```python
from build123d import *

# Parameters (mm, degrees)
SKETCH_1_R          = 1
EXTRUDE_1_DEPTH     = 1.6
SKETCH_2_W          = 16
SKETCH_2_H          = 8
CUT_EXTRUDE_1_DEPTH = 1.6
EXTRUDE_2_DEPTH     = 1.6
SKETCH_4_W          = 1.78
SKETCH_4_H          = 8.1
CUT_EXTRUDE_2_DEPTH = 0.1
CUT_EXTRUDE_START   = 1.6
SKETCH_5_W          = 1.78
SKETCH_5_H          = 8.1
CUT_EXTRUDE_3_DEPTH = 0.1


with BuildPart() as part:
    # 草图1 → 凸台-拉伸1 (new body)
    with BuildSketch(Plane.XY):
        with BuildLine():
            Line((-14, 30), (14, 30))
            ThreePointArc((14, 30), (15.414213562, 29.414213562), (16, 28))
            Line((16, 28), (16, -28))
            ThreePointArc((16, -28), (15.414213562, -29.414213562), (14, -30))
            Line((14, -30), (-14, -30))
            ThreePointArc((-14, -30), (-15.414213562, -29.414213562), (-16, -28))
            Line((-16, -28), (-16, 28))
            ThreePointArc((-16, 28), (-15.414213562, 29.414213562), (-14, 30))
        make_face()
        with Locations((-14, 28)):
            Circle(SKETCH_1_R, mode=Mode.SUBTRACT)
        with Locations((14, 28)):
            Circle(SKETCH_1_R, mode=Mode.SUBTRACT)
    extrude(amount=EXTRUDE_1_DEPTH)

    # 草图2 → 切除-拉伸1 (cut)
    with BuildSketch(Plane.XY):
        with Locations((0, -26)):
            Rectangle(SKETCH_2_W, SKETCH_2_H)
    extrude(amount=CUT_EXTRUDE_1_DEPTH, mode=Mode.SUBTRACT)

    # 草图3 → 凸台-拉伸2 (add)
    with BuildSketch(Plane.XY):
        with BuildLine():
            Line((-13.97, 30), (13.97, 30))
            Line((13.97, 30), (13.97, 39.42))
            ThreePointArc((13.97, 39.42), (13.530660172, 40.480660172), (12.47, 40.92))
            Line((12.47, 40.92), (-12.47, 40.92))
            ThreePointArc((-12.47, 40.92), (-13.530660172, 40.480660172), (-13.97, 39.42))
            Line((-13.97, 39.42), (-13.97, 30))
        make_face()
    extrude(amount=EXTRUDE_2_DEPTH)

    # 草图4 → 切除-拉伸2 (cut)
    with BuildSketch(Plane.XY):
        with Locations((-1.27, 36.37)):
            Rectangle(SKETCH_4_W, SKETCH_4_H)
        with Locations((-3.81, 36.37)):
            Rectangle(SKETCH_4_W, SKETCH_4_H)
        with Locations((-6.35, 36.37)):
            Rectangle(SKETCH_4_W, SKETCH_4_H)
        with Locations((-8.89, 36.37)):
            Rectangle(SKETCH_4_W, SKETCH_4_H)
        with Locations((-11.43, 36.37)):
            Rectangle(SKETCH_4_W, SKETCH_4_H)
        with Locations((11.43, 36.37)):
            Rectangle(SKETCH_4_W, SKETCH_4_H)
        with Locations((8.89, 36.37)):
            Rectangle(SKETCH_4_W, SKETCH_4_H)
        with Locations((6.35, 36.37)):
            Rectangle(SKETCH_4_W, SKETCH_4_H)
        with Locations((3.81, 36.37)):
            Rectangle(SKETCH_4_W, SKETCH_4_H)
        with Locations((1.27, 36.37)):
            Rectangle(SKETCH_4_W, SKETCH_4_H)
    extrude(amount=CUT_EXTRUDE_2_DEPTH, mode=Mode.SUBTRACT)

    # 草图5 → 切除-拉伸3 (cut)
    with BuildSketch(Plane.XY.offset(CUT_EXTRUDE_START)):
        with Locations((-3.81, 36.37)):
            Rectangle(SKETCH_5_W, SKETCH_5_H)
        with Locations((-1.27, 36.37)):
            Rectangle(SKETCH_5_W, SKETCH_5_H)
        with Locations((-11.43, 36.37)):
            Rectangle(SKETCH_5_W, SKETCH_5_H)
        with Locations((-8.89, 36.37)):
            Rectangle(SKETCH_5_W, SKETCH_5_H)
        with Locations((-6.35, 36.37)):
            Rectangle(SKETCH_5_W, SKETCH_5_H)
        with Locations((1.27, 36.37)):
            Rectangle(SKETCH_5_W, SKETCH_5_H)
        with Locations((3.81, 36.37)):
            Rectangle(SKETCH_5_W, SKETCH_5_H)
        with Locations((6.35, 36.37)):
            Rectangle(SKETCH_5_W, SKETCH_5_H)
        with Locations((8.89, 36.37)):
            Rectangle(SKETCH_5_W, SKETCH_5_H)
        with Locations((11.43, 36.37)):
            Rectangle(SKETCH_5_W, SKETCH_5_H)
    extrude(amount=-CUT_EXTRUDE_3_DEPTH, mode=Mode.SUBTRACT)


solid = part.part
```
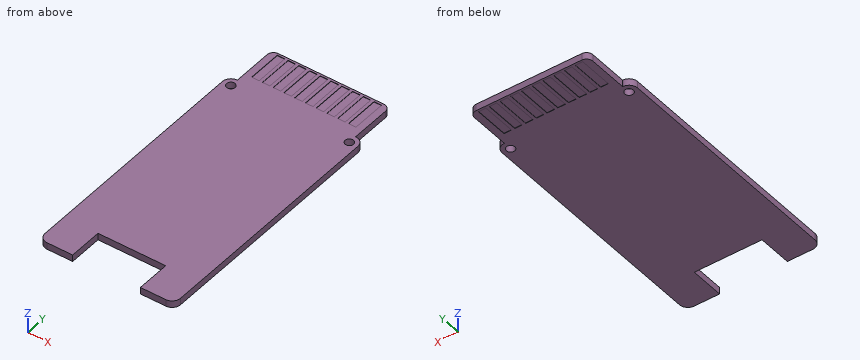
Can you work these out from the model? Positions are in its coordinate system, mm. Coordinates: 2 decimals unless noted, no trailing zeros. Put each result on its own line as item: value. Start each with the question number.
(1) Will this pin go through, and if not, where does the flat tip stop? pin 1 Ø0.9 at (x, y) = (8.5, 37.5) entering from +Z.
(2) Imagine slicing it at A-A on z = 1.1. Give the number of separate pieces and of enclosed holes in the cut face, and give its area (3 significant figures).
(3) I need wall thicknesses on probe 1 along Y at (x, z) = (14, 1); probe 2 along Y at (x, z) = (6.5, 1.2); probe 3 along X at (y, z) = (30.5, 0.5). Which ranges of each line are inside material? Lowest first, please.
Worked answers:
1. pin 1: stops at z = 1.5
2. separate pieces: 1
2. enclosed holes: 2
2. area: 2,090 mm2
3. probe 1: y = -30 to 27, 29 to 30
3. probe 2: y = -22 to 40.92
3. probe 3: x = -13.97 to 13.97
